```python
from build123d import *

# Parameters (mm, degrees)
TOP_EDGE_OUTLINE_W  = 86.5
TOP_EDGE_OUTLINE_H  = 39.5
TOP_EDGE_DEPTH      = 3
TOP_EDGE_DRAFT      = 45
SKETCH13_W          = 72
SKETCH13_H          = 25
DISPLAY_HOLE_DEPTH  = 6
SKETCH14_W          = 92.5
SKETCH14_H          = 45.5
SKETCH14_W_2        = 89.5
SKETCH14_H_2        = 42.5
BOSS_EXTRUDE5_DEPTH = 5
SKETCH15_W          = 128.5
SKETCH15_H          = 45.5
SKETCH15_W_2        = 89.5
SKETCH15_H_2        = 42.5
BOSS_EXTRUDE6_DEPTH = 2
SKETCH16_W          = 128.5
SKETCH16_H          = 45.5
SKETCH16_W_2        = 125.5
SKETCH16_H_2        = 42.5
BOSS_EXTRUDE7_DEPTH = 37
LOFT2_OUTLINE_W     = 33
LOFT2_OUTLINE_H     = 42.5
LOFT2_DEPTH         = 1.5
LOFT2_DRAFT         = 45
SKETCH19_R          = 2.75
SKETCH19_R_2        = 2
BOSS_EXTRUDE8_DEPTH = 1
CUT_EXTRUDE3_START  = -11
SKETCH20_R          = 2
CUT_EXTRUDE3_DEPTH  = 11
SKETCH21_W          = 12
SKETCH21_H          = 8
CUT_EXTRUDE4_DEPTH  = 11
SKETCH22_W          = 4
SKETCH22_H          = 15
BOSS_EXTRUDE9_DEPTH = 3
SKETCH24_W          = 42.5
SKETCH24_H          = 37
CUT_EXTRUDE5_DEPTH  = 17


# Read off the part's stored shape, not the designer's step: Top Edge, Loft2
with BuildPart() as part:
    # Top Edge outline → Top Edge (with draft: the straight prism first)
    with BuildSketch(Plane(origin=(0, 0, 0), x_dir=(1, 0, 0), z_dir=(0, 1, 0))):
        with Locations((0.25, -0.25)):
            Rectangle(TOP_EDGE_OUTLINE_W, TOP_EDGE_OUTLINE_H)
    extrude(amount=-TOP_EDGE_DEPTH)
    # Top Edge: the draft: its side faces are tilted about the plane it starts from
    top_edge_sides = [part.faces().sort_by_distance(p)[0] for p in [
        (-43, -1.5, 0.25),
        (0.25, -1.5, 20),
        (43.5, -1.5, 0.25),
        (0.25, -1.5, -19.5),
    ]]
    draft(top_edge_sides, Plane(origin=(0, 0, 0), x_dir=(1, 0, 0), z_dir=(0, 1, 0)), TOP_EDGE_DRAFT)

    # Sketch13 → Display Hole (cut)
    with BuildSketch(Plane(origin=(0, 0, 0), x_dir=(1, 0, 0), z_dir=(0, 1, 0))):
        Rectangle(SKETCH13_W, SKETCH13_H)
    extrude(amount=-DISPLAY_HOLE_DEPTH, mode=Mode.SUBTRACT)

    # Sketch14 → Boss-Extrude5 (add)
    with BuildSketch(Plane.XZ.offset(3)):
        with Locations((0.25, 0.25)):
            Rectangle(SKETCH14_W, SKETCH14_H)
        with Locations((0.25, 0.25)):
            Rectangle(SKETCH14_W_2, SKETCH14_H_2, mode=Mode.SUBTRACT)
    extrude(amount=BOSS_EXTRUDE5_DEPTH)

    # Sketch15 → Boss-Extrude6 (add)
    with BuildSketch(Plane.XZ.offset(8)):
        with Locations((18.25, 0.25)):
            Rectangle(SKETCH15_W, SKETCH15_H)
        with Locations((0.25, 0.25)):
            Rectangle(SKETCH15_W_2, SKETCH15_H_2, mode=Mode.SUBTRACT)
    extrude(amount=BOSS_EXTRUDE6_DEPTH)

    # Sketch16 → Boss-Extrude7 (add)
    with BuildSketch(Plane.XZ.offset(10)):
        with Locations((18.25, 0.25)):
            Rectangle(SKETCH16_W, SKETCH16_H)
        with Locations((18.25, 0.25)):
            Rectangle(SKETCH16_W_2, SKETCH16_H_2, mode=Mode.SUBTRACT)
    extrude(amount=BOSS_EXTRUDE7_DEPTH)


with BuildPart() as loft2_tool:
    # Loft2 outline → Loft2 (with draft: the straight prism first)
    with BuildSketch(Plane(origin=(0, -6.5, 0), x_dir=(1, 0, 0), z_dir=(0, 1, 0))):
        with Locations((64.5, -0.25)):
            Rectangle(LOFT2_OUTLINE_W, LOFT2_OUTLINE_H)
    extrude(amount=-LOFT2_DEPTH)
    # Loft2: the draft: its side faces are tilted about the plane it starts from
    loft2_sides = [loft2_tool.faces().sort_by_distance(p)[0] for p in [
        (81, -7.25, 0.25),
        (64.5, -7.25, -21),
        (48, -7.25, 0.25),
        (64.5, -7.25, 21.5),
    ]]
    draft(loft2_sides, Plane(origin=(0, -6.5, 0), x_dir=(1, 0, 0), z_dir=(0, 1, 0)), LOFT2_DRAFT)


with BuildPart() as part_1:
    add(part.part)

    # Loft2: add loft2_tool
    add(loft2_tool.part)

    # Sketch19 → Boss-Extrude8 (add)
    with BuildSketch(Plane(origin=(0, -6.5, 0), x_dir=(1, 0, 0), z_dir=(0, 1, 0))):
        with Locations(Location((64.5, 3, 0), (0, 0, 270))):
            Circle(SKETCH19_R)
        with Locations(Location((64.5, 3, 0), (0, 0, 270))):
            Circle(SKETCH19_R_2, mode=Mode.SUBTRACT)
    extrude(amount=BOSS_EXTRUDE8_DEPTH)

    # Sketch20 → Cut-Extrude3 (cut)
    with BuildSketch(Plane(origin=(0, -6.5, 0), x_dir=(1, 0, 0), z_dir=(0, 1, 0)).offset(CUT_EXTRUDE3_START)):
        with Locations(Location((64.5, 3, 0), (0, 0, 90))):
            Circle(SKETCH20_R)
    extrude(amount=CUT_EXTRUDE3_DEPTH, mode=Mode.SUBTRACT)

    # Sketch21 → Cut-Extrude4 (cut)
    with BuildSketch(Plane(origin=(82.5, 0, 0), x_dir=(0, 0, -1), z_dir=(1, 0, 0))):
        with Locations((0, -43)):
            Rectangle(SKETCH21_W, SKETCH21_H)
    extrude(amount=-CUT_EXTRUDE4_DEPTH, mode=Mode.SUBTRACT)

    # Sketch22 → Boss-Extrude9 (add)
    with BuildSketch(Plane.XZ.offset(3)):
        with Locations((-38, 0)):
            Rectangle(SKETCH22_W, SKETCH22_H)
    extrude(amount=BOSS_EXTRUDE9_DEPTH)

    # Sketch24 → Cut-Extrude5 (cut)
    with BuildSketch(Plane.ZY.offset(-81)):
        with Locations((0.25, -28.5)):
            Rectangle(SKETCH24_W, SKETCH24_H)
    extrude(amount=-CUT_EXTRUDE5_DEPTH, mode=Mode.SUBTRACT)


solid = part_1.part
```
For this review, take the finished solid that the model builds, in its own axes (mm). A direction names the side the tool comes from. Round coordinates to 2 decimals unless told otherwise and drop trailing zeros. Write each loop counter-clockwise with the first axis right and the second up, starting at its lowest first coordinate (ties: lowest second). Pieces come first, ordered by that corner, then holes. Notation, with made-up numbers: (27, 72.25) -> (41, 72.25) arc R30 ccw to (41, 110.25) -> close; hole circle Ø2 at (85, 10.25). An arc over 180 degrees is marked (long way). One line per question, with ' | ' between items. Start each with the question number.
(1) Add section D-D, the plane x = 73. Write out the cut boundary in (y, z).
(2) For line 1 along X through (y, z) = (-8.7, -3); line 2 along Z through (x, y) = (-12, -29); line 3 along X through (y, z) = (-7.65, -3), list the stretches that pass through material, from the lowest coordinate up. Write a range as from..to.
(3) Mouldability with a two-part tool opening along Z and no side actions: class faces 6 (the face through (-0.4, -1.5, -21)), 7 (the face through (67.227, -6.007, -3.358)), 8 (the face through (18, -25, -21)), 9 (the face through (82.5, -9, 0)) as released by +Z, released by -Z, zero draft, split by the parting line, or undercut.
(4) Tool access review of faces 1 (the face through (-36, -2, 0)), 2 (the face through (0, 0, -13)), 3 (the face through (-40, -4, 0)), 4 (the face through (18, -47, 22)), 5 (the face through (62, -5.5, -3)): name each direction out of +Z, -Z, +X, -X, +Y, -Y from which nothing blocks a thin tool from reaching the whole face with its end or side.
(5) Add section A-A, the plane x = 11. Write out the cut boundary in (y, z), plus the area to 4 significant figures.
(6) Insertion check: P1, Ø16.5, axis at x = 57.5, z = 0.5, coming from the +Y side; P2, Ø2.5, axis at x = 2.5, y = -1.5, coming from the -Z side; P3, Ø10, axis at x = -33, z = 1, coming from the -Y side; P4, Ø1.6, axis at x = 65, z = -4, coming from the +Y side. Each pin has a flat end and moves straight along its axis. Give the tip position at first contact, or say it passes through.
(7) Add section B-B, the plane z = -3. Write out the cut boundary in (x, y).
(8) Add section C-C, the plane y = -30. Write out the cut boundary in (x, z), plus the area to 3 significant figures.
Answer list:
1) outline: (-47, -22.5) -> (-8, -22.5) -> (-6.5, -21) -> (-6.5, 21.5) -> (-8, 23) -> (-47, 23) -> (-47, 21.5) -> (-10, 21.5) -> (-10, -21) -> (-47, -21) -> close
2) line 1: -46..-44.5, 45..62.5, 66.5..82.5 | line 2: -22.5..-21, 21.5..23 | line 3: -46..-44.5, 45..46.5, 46.85..62.5, 66.5..82.15
3) face 6: released by -Z | face 7: split by the parting line | face 8: undercut | face 9: zero draft
4) face 1: +Y, -Y | face 2: +Z, -Z, +X, -X, +Y | face 3: -Y | face 4: +Z, -Z, +X, -X, -Y | face 5: +Z, -Z, +X, +Y
5) outline: (-47, -22.5) -> (-3, -22.5) -> (0, -19.5) -> (0, -12.5) -> (-3, -12.5) -> (-3, -21) -> (-47, -21) -> close; (-47, 21.5) -> (-3, 21.5) -> (-3, 12.5) -> (0, 12.5) -> (0, 20) -> (-3, 23) -> (-47, 23) -> close | area: 184.5 mm²
6) P1: y = -5.5 | P2: z = -22.25 | P3: y = -6 | P4: through
7) outline: (-46, -47) -> (-44.5, -47) -> (-44.5, -3) -> (-40, -3) -> (-40, -6) -> (-36, -6) -> (-36, 0) -> (-43, 0) -> (-46, -3) -> close; (36, -3) -> (45, -3) -> (45, -10) -> (62.5, -10) -> (62.5, -5.5) -> (61.75, -5.5) -> (61.75, -6.5) -> (48, -6.5) -> (46.5, -8) -> (46.5, -3) -> (43.5, 0) -> (36, 0) -> close; (66.5, -10) -> (82.5, -10) -> (82.5, -8) -> (81, -6.5) -> (67.25, -6.5) -> (67.25, -5.5) -> (66.5, -5.5) -> close
8) outline: (-46, -22.5) -> (82.5, -22.5) -> (82.5, -21) -> (-44.5, -21) -> (-44.5, 21.5) -> (82.5, 21.5) -> (82.5, 23) -> (-46, 23) -> close | area: 449 mm²
